Geometry: final body of the model. Coordinates: model frame, mm. Give positions to 0.01 mm unless a question says otherwise; leave off trailing zeros. Loops run counter-clockwise (first coordinate to the right, second up) from the corner with the lowest first, then second, coordinate; pieces in that order, holes last. Notation, with made-up numbers: (88.5, -3) -> (124.5, -3) arc R28 cw to (124.5, 26) -> close; hole circle Ø2 at (83, 80.25). An arc over 180 degrees is marked (long way). Answer in a Markdown table with one row per item. Add a question column.
1) Section query A-A (z = 0). Return the cut outline in (x, y).
2) Line query: line 1 (Y direction, x = -0.5, z = 0); line 2 (Z direction, x = 0, y = -30); line 3 (Y direction, x = 1.75, z = -2.5). Output: solid intervals per line, ascending. Write a range as from..to.
3) Section query D-D (x = 1). Give the number of separate pieces and of enclosed holes in the cut face, plus the area to 3 significant figures.
4) Section query C-C (y = 18). Return the cut outline in (x, z), plus the area to 3 significant figures.
5) First-contact query: P1, Ø4, axis at x = -3, y = 19.5, coming from the +Z side. Flat tip, straight axial feed; report the tip coordinate or a pass-through.
6) Section query B-B (y = -30). Return the cut outline in (x, z), plus the area to 3 significant figures.
7) Draft query along Z for faces 1 (the cylindrical face through (-0.08, 32.03, 2.21)), 2 (the cylindrical face through (0, 1, 8)), 3 (the flat face through (0, -37.5, 0)). Return one class per face: +Z half, -Z half, draft (parallel to the pull), parting line (faces both ways), or undercut.
```python
from build123d import *

# Parameters (mm, degrees)
EXTRUDE_1_DEPTH          = 37.5
CUT_EXTRUDE_1_DEPTH      = 39.810570802
CUT_EXTRUDE_1_DEPTH_BACK = 39.810570802
SKETCH_2_R               = 3
FILLET_2_R               = 1


with BuildPart() as part:
    # 草图1 → 凸台-拉伸1 (new, symmetric)
    with BuildSketch(Plane(origin=(0, 0, 0), x_dir=(1, 0, 0), z_dir=(0, 1, 0))):
        with BuildLine():
            Line((-6, -7.350239011), (-6, 7.350239011))
            ThreePointArc((-6, 7.350239011), (0, 5.999349652), (6, 7.350239011))
            Line((6, 7.350239011), (6, -7.350239011))
            ThreePointArc((6, -7.350239011), (0, -8.000650348), (-6, -7.350239011))
        make_face()
    extrude(amount=EXTRUDE_1_DEPTH, both=True)

    # 草图2 → 切除-拉伸1 (cut, two sides: drawn at the far end of the back side and taken through both)
    with BuildSketch(Plane(origin=(0, 0, 0), x_dir=(0, 0, -1), z_dir=(1, 0, 0)).offset(-CUT_EXTRUDE_1_DEPTH_BACK)):
        with Locations((0, 30)):
            Circle(SKETCH_2_R)
        with Locations((0, -30)):
            Circle(SKETCH_2_R)
    extrude(amount=CUT_EXTRUDE_1_DEPTH + CUT_EXTRUDE_1_DEPTH_BACK, mode=Mode.SUBTRACT)

    # 圆角2
    fillet_2_edges = [part.edges().sort_by_distance(p)[0] for p in [
        (0, 37.5, -5.999349652),
        (-6, 37.5, 0),
        (0, 37.5, 8.000650348),
        (-6, -37.5, 0),
        (0, -37.5, -5.999349652),
        (6, -37.5, 0),
        (0, -37.5, 8.000650348),
        (-6, 0, 7.350239011),
        (-6, 0, -7.350239011),
        (6, 0, -7.350239011),
        (6, 0, 7.350239011),
        (6, 37.5, 0),
    ]]
    fillet(fillet_2_edges, radius=FILLET_2_R)


solid = part.part
```
Evaluation:
| question | item | result |
|---|---|---|
| 1 | outline | (-6, -36.5) arc R1 ccw to (-5, -37.5) -> (5, -37.5) arc R1 ccw to (6, -36.5) -> (6, -33) -> (-6, -33) -> close; (-6, -27) -> (6, -27) -> (6, 27) -> (-6, 27) -> close; (-6, 33) -> (6, 33) -> (6, 36.5) arc R1 ccw to (5, 37.5) -> (-5, 37.5) arc R1 ccw to (-6, 36.5) -> close |
| 2 | line 1 | -37.5..-33, -27..27, 33..37.5 |
| 2 | line 2 | -6..-3, 3..8 |
| 2 | line 3 | -37.5..-31.66, -28.34..28.34, 31.66..37.5 |
| 3 | separate pieces | 1 |
| 3 | enclosed holes | 2 |
| 3 | area | 994 mm² |
| 4 | outline | (-6, -5.86) arc R1 ccw to (-4.67, -6.8) arc R14 cw to (4.67, -6.8) arc R1 ccw to (6, -5.86) -> (6, 6.53) arc R1 ccw to (5.19, 7.52) arc R28 ccw to (-5.19, 7.52) arc R1 ccw to (-6, 6.53) -> close |
| 4 | area | 169 mm² |
| 5 | P1 | z = 7.98 |
| 6 | outline | (-6, -5.86) arc R1 ccw to (-4.67, -6.8) arc R14 cw to (4.67, -6.8) arc R1 ccw to (6, -5.86) -> (6, -3) -> (-6, -3) -> close; (-6, 3) -> (6, 3) -> (6, 6.53) arc R1 ccw to (5.19, 7.52) arc R28 ccw to (-5.19, 7.52) arc R1 ccw to (-6, 6.53) -> close |
| 6 | area | 97.5 mm² |
| 7 | face 1 | undercut |
| 7 | face 2 | +Z half |
| 7 | face 3 | draft |
